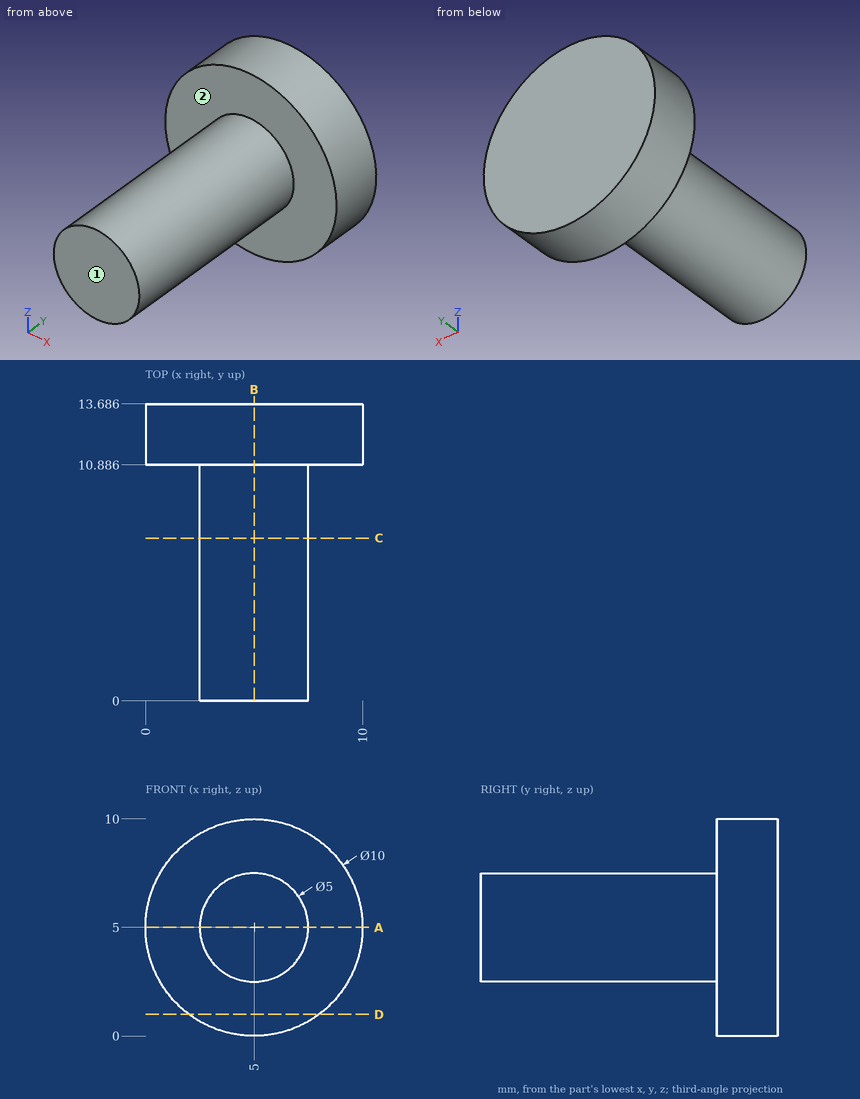
The drawing under review shows one solid part. Ordinate dimensions are in mm from its lowest x, y, z. A direction names the side the tool comes from. Coordinates: 2 decimals unless noted, no trailing zeros. Write each loop counter-clockwise with the first axis right and the second up, starting at its lowest first coordinate (ties: lowest second). Pieces come first, ordered by that corner, then holes.
1) Add section B-B (x = 5). Write out the cut boundary in (y, z), plus the area to 3 significant figures.
2) Add section D-D (z = 1). Write out the cut boundary in (x, y).
3) To check wall thickness, follow L1, parallel to Y at x = 2.5, z = 8.5; L2, parallel to Z at x = 7.25, y = 4.5. State the ranges of each line that lie inside material, in increasing order.
4) Add section A-A (z = 5). Write out the cut boundary in (x, y), plus the area to 3 significant figures.
5) Insertion check: pin 1 (2 mm diameter, centred on y = 2.5, z = 5.5, fed in from +X); pin 2 (2 mm diameter, centred on y = 6.5, z = 3, fed in from +X); pin 3 (1.5 mm diameter, centred on x = 4.5, y = 7, fed in from -Z). Each pin has a flat end and moves straight along its axis. Give the tip position at first contact, or say it passes through.
6) Machinability: for the marked faces 1 and 2, which of the approach directions +Z, -Z, +X, -X, +Y, -Y give a long, thin tool a straight path to every point of the face, cutting with its end or side? Answer none if there is none.
7) Add section C-C (y = 7.5). Write out the cut boundary in (x, z).
Check result:
1. outline: (0, 2.5) - (10.89, 2.5) - (10.89, 0) - (13.69, 0) - (13.69, 10) - (10.89, 10) - (10.89, 7.5) - (0, 7.5) - close
1. area: 82.4 mm2
2. outline: (2, 10.89) - (8, 10.89) - (8, 13.69) - (2, 13.69) - close
3. L1: y = 10.89 to 13.69
3. L2: z = 3.91 to 6.09
4. outline: (0, 10.89) - (2.5, 10.89) - (2.5, 0) - (7.5, 0) - (7.5, 10.89) - (10, 10.89) - (10, 13.69) - (0, 13.69) - close
4. area: 82.4 mm2
5. pin 1: stops at x = 7.5
5. pin 2: stops at x = 7.29
5. pin 3: stops at z = 2.5
6. face 1: +Z, -Z, +X, -X, -Y
6. face 2: -Y
7. outline: circle Ø5 at (5, 5)
